CAD build for the part. Positions are in the model's coordinates, mm. Face numbers are marked on the shaded views. A direction names the side the tool comes from. Coordinates: 2 decimals unless noted, no trailing zeros. Write each loop counter-clockwise with the first axis right and the second up, starting at its lowest first coordinate (ties: lowest second). Pieces come first, ordered by that corner, then holes. Notation, with made-up numbers: (5.25, -6.5) - (16.25, -6.5) arc R26 ccw to (16.25, 9.5) - close; hole circle Ø1 at (89, -15.5). An arc over 180 degrees is marked (long way). Answer in a Markdown table with one row per item. Add a question column.
Q1. 3-axis set-ups, long thin cutter, end or side, ignore diameter. For the marked faces 1 and 2: which of +Z, -Z, +X, -X, +Y, -Y reach the whole face in a straight line?
Q2. Band-saw the part on B-B (y = -25.5). State how many separate pieces and enclosed holes the cut face has, and give its area (3 significant figures).
Q3. Band-saw the part on C-C (x = -126.5). List the corners of the cut face in (y, z), and give its area (3 significant figures).
Q4. Two-plate mould, pull along Y, no slides. Class the marked faces 3, 4 and 5: +Y half, -Y half, draft (parallel to the pull), parting line (faces both ways), or undercut.
Q5. Drill centre lines: line 1 along Y through (x, z) = (-400, 80); line 2 along Y through (x, z) = (-237, 0); line 3 along X through (y, z) = (18, 83.5). Where is each one in solid material? Low to high. Write a range as from..to.
Q6. Band-saw the part on A-A (z = 81). List the corners of the cut face in (x, y), and give its area (3 significant figures).
Q7. Pin check, flat tips, straight feed: pin 1 (8 mm diameter, centred on y = 23.5, z = -58, fed in from +X); pin 2 (1.5 mm diameter, centred on x = -83.5, z = 43, fed in from +Y); pin 3 (8 mm diameter, centred on x = -345, z = 0.5, fed in from +Y). Stop position of each tip, or through.
```python
from build123d import *

# Parameters (mm, degrees)
SKETCH4_R           = 38.155726857
BOSS_EXTRUDE1_DEPTH = 150
SKETCH5_R           = 46
SKETCH5_R_2         = 44.09
CUT_EXTRUDE1_DEPTH  = 140


with BuildPart() as part:
    # Sketch4 → Boss-Extrude1 (new body)
    with BuildSketch(Plane.XY):
        with Locations((-400, 0)):
            Circle(SKETCH4_R)
    extrude(amount=BOSS_EXTRUDE1_DEPTH)

    # Sweep2: sweep along a path in Sketch2
    with BuildLine(Plane(origin=(0, 0, 0), x_dir=(1, 0, 0), z_dir=(0, 1, 0))) as sweep2_path:
        Line((0, 120), (0, 50))
        ThreePointArc((0, 50), (-14.644660941, 14.644660941), (-50, 0))
        Line((-50, 0), (-350, 0))
        ThreePointArc((-350, 0), (-385.355339059, -14.644660941), (-400, -50))
        Line((-400, -50), (-400, -150))
    # Sketch5 → Sweep2 (sweep)
    with BuildSketch(Plane.XY.offset(150)):
        with Locations((-400, 0)):
            Circle(SKETCH5_R)
        with Locations((-400, 0)):
            Circle(SKETCH5_R_2, mode=Mode.SUBTRACT)
    sweep(path=sweep2_path.line)

    # Sketch6 → Cut-Extrude1 (cut)
    with BuildSketch(Plane(origin=(0, 0, 0), x_dir=(-1, 0, 0), z_dir=(0, 0, -1))):
        with BuildLine():
            ThreePointArc((408.740673251, -37.141084033), (438.155726857, 0), (408.740673251, 37.141084033))
            ThreePointArc((408.740673251, 37.141084033), (432.21706088, 0), (408.740673251, -37.141084033))
        make_face()
    extrude(amount=-CUT_EXTRUDE1_DEPTH, mode=Mode.SUBTRACT)


solid = part.part
```
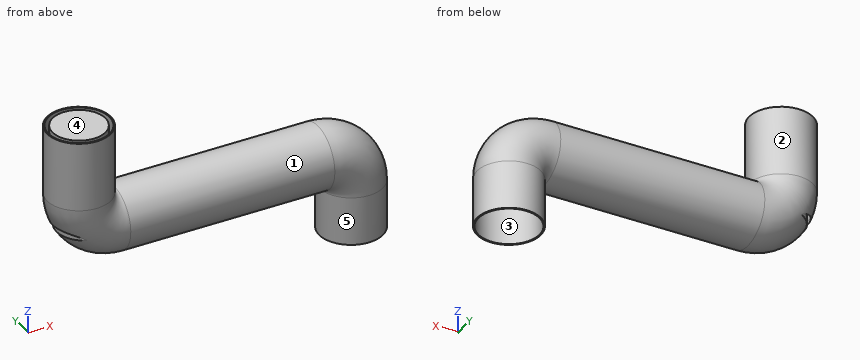
Checked values:
| question | item | result |
|---|---|---|
| 1 | face 1 | none |
| 1 | face 2 | +Z |
| 2 | separate pieces | 3 |
| 2 | enclosed holes | 0 |
| 2 | area | 10,700 mm² |
| 3 | outline | circle Ø92 at (0, 0); hole circle Ø88.18 at (0, 0) |
| 3 | area | 541 mm² |
| 4 | face 3 | undercut |
| 4 | face 4 | draft |
| 4 | face 5 | parting line |
| 5 | line 1 | y = -46..-44.09, -38.16..38.16, 44.09..46 |
| 5 | line 2 | y = -46..-44.09, 44.09..46 |
| 5 | line 3 | x = -442.33..-440.25, -428.07..-366.36, -359.75..-357.67 |
| 6 | outline | circle Ø92 at (-400, 0); (-408.74, -37.14) arc R38.16 ccw (long way) to (-408.74, 37.14) arc R41.12 ccw to start; hole circle Ø88.18 at (-400, 0) |
| 6 | area | 4,740 mm² |
| 7 | pin 1 | stops at x = 41.66 |
| 7 | pin 2 | stops at y = 18.19 |
| 7 | pin 3 | stops at y = 46 |
